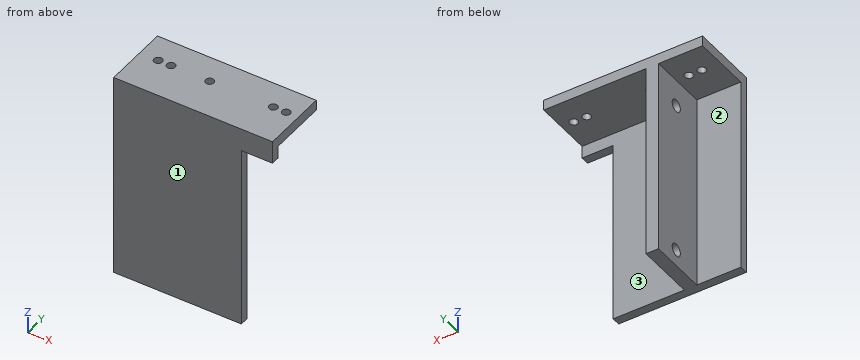
from build123d import *

# Parameters (mm, degrees)
SKETCH1_W                = 50
SKETCH1_H                = 16.1
BOSS_EXTRUDE1_DEPTH      = 3
SKETCH3_R                = 1.5
CUT_EXTRUDE1_DEPTH       = 4
SKETCH4_W                = 2.5
SKETCH4_H                = 16.1
BOSS_EXTRUDE2_DEPTH      = 35.4
BOSS_EXTRUDE2_DEPTH_BACK = 13.6
SKETCH6_R                = 1
CUT_EXTRUDE2_DEPTH       = 45
SKETCH10_W               = 49
SKETCH10_H               = 2
BOSS_EXTRUDE4_DEPTH      = 47.5
CUT_EXTRUDE5_DEPTH       = 15.1
CUT_EXTRUDE5_DEPTH_BACK  = 3


with BuildPart() as part:
    # Sketch1 → Boss-Extrude1 (new body)
    with BuildSketch(Plane(origin=(0, 0, 0), x_dir=(0, 0, -1), z_dir=(1, 0, 0))):
        with Locations((25, 8.05)):
            Rectangle(SKETCH1_W, SKETCH1_H)
    extrude(amount=BOSS_EXTRUDE1_DEPTH)

    # Sketch3 → Cut-Extrude1 (cut, through all)
    with BuildSketch(Plane(origin=(3, 0, 0), x_dir=(0, 0, -1), z_dir=(1, 0, 0))):
        with Locations((46, 9.55)):
            Circle(SKETCH3_R)
        with Locations((9, 9.55)):
            Circle(SKETCH3_R)
    extrude(amount=-CUT_EXTRUDE1_DEPTH, mode=Mode.SUBTRACT)

    # Sketch4 → Boss-Extrude2 (add, two sides)
    with BuildSketch(Plane(origin=(3, 0, 0), x_dir=(0, 0, -1), z_dir=(1, 0, 0))) as boss_extrude2_sk:
        with Locations((1.25, 8.05)):
            Rectangle(SKETCH4_W, SKETCH4_H)
    extrude(amount=BOSS_EXTRUDE2_DEPTH)
    extrude(boss_extrude2_sk.sketch, amount=-BOSS_EXTRUDE2_DEPTH_BACK)

    # Sketch6 → Cut-Extrude2 (cut)
    with BuildSketch(Plane(origin=(0, 0, -2.5), x_dir=(-1, 0, 0), z_dir=(0, 0, -1))):
        with Locations((6.15, 9.55)):
            Circle(SKETCH6_R)
        with Locations((3.05, 9.55)):
            Circle(SKETCH6_R)
        with Locations((-6.25, 9.55)):
            Circle(SKETCH6_R)
        with Locations((-21.55, 9.55)):
            Circle(SKETCH6_R)
        with Locations((-24.65, 9.55)):
            Circle(SKETCH6_R)
    extrude(amount=-CUT_EXTRUDE2_DEPTH, mode=Mode.SUBTRACT)

    # Sketch10 → Boss-Extrude4 (add)
    with BuildSketch(Plane(origin=(0, 0, -2.5), x_dir=(-1, 0, 0), z_dir=(0, 0, -1))):
        with Locations((-13.9, 1)):
            Rectangle(SKETCH10_W, SKETCH10_H)
    extrude(amount=BOSS_EXTRUDE4_DEPTH)

    # Sketch13 → Cut-Extrude5 (cut, two sides)
    with BuildSketch(Plane(origin=(0, 2, 0), x_dir=(1, 0, 0), z_dir=(0, 1, 0))) as cut_extrude5_sk:
        Polygon((20.1, 5.5), (20.1, 50), (38.4, 50), (38.4, 0), (27.6, 0), (27.6, 5.5), align=None)
    extrude(amount=CUT_EXTRUDE5_DEPTH, mode=Mode.SUBTRACT)
    extrude(cut_extrude5_sk.sketch, amount=-CUT_EXTRUDE5_DEPTH_BACK, mode=Mode.SUBTRACT)


solid = part.part
Can you work these out from the model? Positions are in its coordinate system, mm. Face numbers are marked on the shaded views. A direction names the side the tool comes from. Coordinates: 2 decimals unless noted, no trailing zeros. Order: outer loops, then holes, each group sorted by start corner. A loop starts at its lowest first (then second) coordinate and runs counter-clockwise, first axis right, second up. Notation, with made-up numbers: M -18.5,-13.75 L 35.5,-13.75 A32 ccw 35.5,14.25 Z; hole C -16.5,-15 d4. An arc over 180 degrees is marked long. Answer as CSV lines item,"result".
(1) Suppose I cut it at C-C on y = 13.25. Please give me the cut outline in (x, z).
Geometry check:
outline,"M -10.6,-2.5 L 0,-2.5 L 0,-50 L 3,-50 L 3,-2.5 L 27.6,-2.5 L 27.6,0 L -10.6,0 Z"
(2) Suppose I cut it at D-D on z = -36. Please give me the cut outline in (x, y), plus the area to 3 significant figures.
Geometry check:
outline,"M -10.6,0 L 20.1,0 L 20.1,2 L 3,2 L 3,16.1 L 0,16.1 L 0,2 L -10.6,2 Z"
area,"104 mm^2"
(3) Suppose I cut it at B-B on z = -9. Please give me the cut outline in (x, y).
Geometry check:
outline,"M -10.6,0 L 20.1,0 L 20.1,2 L 3,2 L 3,8.05 L 0,8.05 L 0,2 L -10.6,2 Z; M 0,11.05 L 3,11.05 L 3,16.1 L 0,16.1 Z"
(4) Suppose I cut it at A-A on x = 24.65. Please give me the cut outline in (y, z), plus the area to 4 significant figures.
Geometry check:
outline,"M 0,-5.5 L 2,-5.5 L 2,-2.5 L 8.55,-2.5 L 8.55,0 L 0,0 Z; M 10.55,-2.5 L 16.1,-2.5 L 16.1,0 L 10.55,0 Z"
area,"41.25 mm^2"
(5) Please list where these lines run through material, in increasing order: L1, parallel to Y at x = 6.25, z = -1.95; L2, parallel to Y at x = 2.05, z = -9; L3, parallel to Z at x = -7.5, y = 12.25.
Geometry check:
L1,"0 to 8.55, 10.55 to 16.1"
L2,"0 to 8.05, 11.05 to 16.1"
L3,"-2.5 to 0"
(6) I'm going to push flat-ended pins straight in: pin 1 (4 mm diameter, centred on x = 13.5, y = 8, fed in from -Z); pin 2 (2.5 mm diameter, centred on y = 9.55, z = -9, fed in from -X); pin 3 (3 mm diameter, centred on y = 12, z = -32, fed in from +X); pin 4 (8.5 mm diameter, centred on x = -6.5, z = -31, fed in from +Y). Where does each tip first touch, or does it pass through?
Geometry check:
pin 1,"z = -2.5"
pin 2,"through"
pin 3,"x = 3"
pin 4,"y = 2"
(7) On a 3-axis mill with a long thin cutter (end or side, diameter ignored), from which of +Z, -Z, +X, -X, +Y, -Y can I reach the whole of each face in a straight line? I mean the marked faces 1, 2 and 3. Say none if no direction works.
Geometry check:
face 1,"+Z, -Z, +X, -X, -Y"
face 2,"-Z, -X, +Y"
face 3,"-Z, +X, +Y"
